from build123d import *

# Parameters (mm, degrees)
SKETCH1_W           = 65.4
SKETCH1_H           = 65.4
BOSS_EXTRUDE1_DEPTH = 1.12
FILLET1_R           = 4
BOSS_EXTRUDE2_START = 10
BOSS_EXTRUDE2_DEPTH = 10
CUT_EXTRUDE1_REACH  = 75.96
SKETCH4_W           = 19.5
SKETCH4_H           = 3.5
CUT_EXTRUDE2_DEPTH  = 2.5
FILLET3_R           = 2
SKETCH5_W           = 1.6
SKETCH5_H           = 49.8
SKETCH5_W_2         = 49.8
SKETCH5_H_2         = 1.6
BOSS_EXTRUDE3_DEPTH = 1
BOSS_EXTRUDE4_DEPTH = 3.8
SKETCH7_R           = 1.4
CUT_EXTRUDE3_DEPTH  = 11.12
SKETCH8_R           = 2.75
CUT_EXTRUDE4_DEPTH  = 4
FILLET4_R           = 1.5
FILLET5_R           = 1.5


with BuildPart() as part:
    # Sketch1 → Boss-Extrude1 (new body)
    with BuildSketch(Plane(origin=(0, 0, 0), x_dir=(1, 0, 0), z_dir=(0, 1, 0))):
        Rectangle(SKETCH1_W, SKETCH1_H)
    extrude(amount=BOSS_EXTRUDE1_DEPTH)

    # Fillet1
    fillet1_edges = [part.edges().sort_by_distance(p)[0] for p in [
        (32.7, 0.56, 32.7),
        (-32.7, 0.56, 32.7),
        (-32.7, 0.56, -32.7),
        (32.7, 0.56, -32.7),
    ]]
    fillet(fillet1_edges, radius=FILLET1_R)

    # Sketch2 → Boss-Extrude2 (add)
    with BuildSketch(Plane(origin=(0, 1.12, 0), x_dir=(1, 0, 0), z_dir=(0, 1, 0)).offset(BOSS_EXTRUDE2_START)):
        with BuildLine():
            Line((-32.7, 28.7), (-32.7, -28.7))
            ThreePointArc((-32.7, -28.7), (-31.528427125, -31.528427125), (-28.7, -32.7))
            Line((-28.7, -32.7), (28.7, -32.7))
            ThreePointArc((28.7, -32.7), (31.528427125, -31.528427125), (32.7, -28.7))
            Line((32.7, -28.7), (32.7, 28.7))
            ThreePointArc((32.7, 28.7), (31.528427125, 31.528427125), (28.7, 32.7))
            Line((28.7, 32.7), (-28.7, 32.7))
            ThreePointArc((-28.7, 32.7), (-31.528427125, 31.528427125), (-32.7, 28.7))
        make_face()
        with BuildLine():
            Line((24.9, 28.7), (-24.9, 28.7))
            ThreePointArc((-24.9, 28.7), (-26.012994231, 26.012994231), (-28.7, 24.9))
            Line((-28.7, 24.9), (-28.7, -24.9))
            ThreePointArc((-28.7, -24.9), (-26.012994231, -26.012994231), (-24.9, -28.7))
            Line((-24.9, -28.7), (24.9, -28.7))
            ThreePointArc((24.9, -28.7), (26.012994231, -26.012994231), (28.7, -24.9))
            Line((28.7, -24.9), (28.7, 24.9))
            ThreePointArc((28.7, 24.9), (26.012994231, 26.012994231), (24.9, 28.7))
        make_face(mode=Mode.SUBTRACT)
    extrude(amount=-BOSS_EXTRUDE2_DEPTH)

    # Sketch3 → Cut-Extrude1 (cut, up to next)
    with BuildSketch(Plane(origin=(0, 0, -32.7), x_dir=(-1, 0, 0), z_dir=(0, 0, -1)), mode=Mode.PRIVATE) as cut_extrude1_sk1:
        with BuildLine():
            Line((-3, 6.5), (3, 6.5))
            ThreePointArc((3, 6.5), (5, 4.5), (3, 2.5))
            Line((3, 2.5), (-3, 2.5))
            ThreePointArc((-3, 2.5), (-5, 4.5), (-3, 6.5))
        make_face()
    cut_extrude1_tool1 = extrude(cut_extrude1_sk1.sketch, amount=-CUT_EXTRUDE1_REACH, mode=Mode.PRIVATE) & part.part
    add(cut_extrude1_tool1.solids().sort_by_distance((0, 4.5, -32.7))[0], mode=Mode.SUBTRACT)

    # Sketch4 → Cut-Extrude2 (cut)
    with BuildSketch(Plane.XY.offset(-28.7)):
        with Locations((0, 2.87)):
            Rectangle(SKETCH4_W, SKETCH4_H)
    extrude(amount=-CUT_EXTRUDE2_DEPTH, mode=Mode.SUBTRACT)

    # Fillet3
    # the kernel refuses this fillet: 2 mm, written as the material it takes off along each edge
    with BuildSketch(Plane(origin=(-0.003603246, 4.62, -28.7), x_dir=(0, 1, 0), z_dir=(1, 0, 0)), Plane(origin=(-9.75, 4.62, -28.7), x_dir=(0, 1, 0), z_dir=(1, 0, 0))) as fillet3_piece_1:
        with BuildLine():
            CenterArc((FILLET3_R, -FILLET3_R), FILLET3_R, 90, 90)
            Line((0, -FILLET3_R), (0, 0))
            Line((0, 0), (FILLET3_R, 0))
        make_face()
    extrude(amount=9.753603246, mode=Mode.SUBTRACT)

    # Sketch5 → Boss-Extrude3 (add)
    with BuildSketch(Plane(origin=(0, 11.12, 0), x_dir=(1, 0, 0), z_dir=(0, 1, 0))):
        with Locations((-29.5, 0)):
            Rectangle(SKETCH5_W, SKETCH5_H)
        with Locations((0, -29.5)):
            Rectangle(SKETCH5_W_2, SKETCH5_H_2)
        with Locations((29.5, 0)):
            Rectangle(SKETCH5_W, SKETCH5_H)
        with Locations((0, 29.5)):
            Rectangle(SKETCH5_W_2, SKETCH5_H_2)
    extrude(amount=BOSS_EXTRUDE3_DEPTH)

    # Sketch6 → Boss-Extrude4 (add)
    with BuildSketch(Plane(origin=(0, 1.12, 0), x_dir=(1, 0, 0), z_dir=(0, 1, 0))):
        Polygon((-9.5, -4.3), (9.5, -4.3), (9.5, 1.7), (11.5, 1.7), (11.5, -6.3), (-11.5, -6.3), (-11.5, 1.7), (-9.5, 1.7), align=None)
    extrude(amount=BOSS_EXTRUDE4_DEPTH)

    # Sketch7 → Cut-Extrude3 (cut)
    with BuildSketch(Plane(origin=(0, 11.12, 0), x_dir=(1, 0, 0), z_dir=(0, 1, 0))):
        with Locations(Location((-28.9, 28.9, 0), (0, 0, 270))):
            Circle(SKETCH7_R)
        with Locations(Location((28.9, 28.9, 0), (0, 0, 270))):
            Circle(SKETCH7_R)
        with Locations(Location((28.9, -28.9, 0), (0, 0, 270))):
            Circle(SKETCH7_R)
        with Locations(Location((-28.9, -28.9, 0), (0, 0, 270))):
            Circle(SKETCH7_R)
    extrude(amount=-CUT_EXTRUDE3_DEPTH, mode=Mode.SUBTRACT)

    # Sketch8 → Cut-Extrude4 (cut)
    with BuildSketch(Plane.XZ):
        with Locations(Location((-28.9, 28.9, 0), (0, 0, 270))):
            Circle(SKETCH8_R)
        with Locations(Location((28.9, 28.9, 0), (0, 0, 270))):
            Circle(SKETCH8_R)
        with Locations(Location((28.9, -28.9, 0), (0, 0, 270))):
            Circle(SKETCH8_R)
        with Locations(Location((-28.9, -28.9, 0), (0, 0, 270))):
            Circle(SKETCH8_R)
    extrude(amount=-CUT_EXTRUDE4_DEPTH, mode=Mode.SUBTRACT)

    # Fillet4
    fillet4_edges = [part.edges().sort_by_distance(p)[0] for p in [
        (-11.5, 1.12, 2.3),
        (0, 1.12, 6.3),
        (11.5, 1.12, 2.3),
    ]]
    fillet(fillet4_edges, radius=FILLET4_R)

    # Fillet5
    fillet5_edges = [part.edges().sort_by_distance(p)[0] for p in [
        (-17.325, 1.12, -28.7),
        (26.012994231, 1.12, -26.012994231),
        (17.325, 1.12, -28.7),
        (-26.012994231, 1.12, -26.012994231),
        (-28.7, 1.12, 0),
        (-26.012994231, 1.12, 26.012994231),
        (0, 1.12, 28.7),
        (26.012994231, 1.12, 26.012994231),
        (28.7, 1.12, 0),
    ]]
    fillet(fillet5_edges, radius=FILLET5_R)


solid = part.part
Part model, mm, in its own coordinate system. A direction names the side the tool comes from. Coordinates: 2 decimals unless noted, no trailing zeros. Loops run counter-clockwise (first coordinate to the right, second up) from the corner with the lowest first, then second, coordinate; pieces in that order, holes last. Notation, with made-up numbers: (20.25, 81) - (61.25, 81) arc R16 ccw to (61.25, 104) - close; hole circle Ø7 at (70, -30.75). An arc over 180 degrees is marked (long way). Write each question's results on one line, items separated by ' | '. Start each with the question number.
Q1. Which spindle directions (+Z, -Z, +X, -X, +Y, -Y) get a long thin tool onto all of the face, cutting with end or side? Do faces 3 (the cylindrical face through (-4.47, 6.124, -28.763)), 4 (the flat face through (0, 2.5, -32)), 5 (the flat face through (-32.7, 6, 0)), 6 (the flat face through (0, 7, 28.7)), 7 (the cylindrical face through (29.021, 1.972, 31.647)). Say none if no direction does.
Q2. Slice it at B-B on x = 21. Give the cut face in (y, z), and give its area (3 significant figures).
Q3. Probe line 1 along X through (y, z) = (9.5, -28.9) (3 decimals); line 2 along X through (y, z) = (2.6, 28.9) (3 decimals); line 3 along X through (y, z) = (11, 16). List the from-to ranges inside material, lowest first.
Q4. Slice it at C-C on z = -17. Give the cut face in (x, y), and give its area (3 significant figures).
Q5. Slice it at D-D on x = -10.5. Give the cut face in (y, z), and give its area (3 significant figures).
Q6. Two-plate mould, pull along Z, no slides. Class faces 1 (the flat face through (0, 12.12, 29)), 2 (the flat face through (11.5, 4, 2)): +Z half, -Z half, draft (parallel to the pull), parting line (faces both ways), or undercut.
Q7. Slice it at A-A on y = 8.5. Give the cut face in (x, z), and give its area (3 significant figures).
Q8. Drop flat-ended pins along their axis: pin 1 Ø2 at (x, y) = (0.5, 4.5) entering from -Z; pin 2 Ø3 at (x, z) = (-28.9, 28.9) entering from +Y; pin 3 Ø9 at (x, z) = (-4.5, 2) entering from +Y. Give the stop position or say it passes through.
Answer:
1) face 3: none | face 4: -Z | face 5: +Z, -Z, -X, +Y, -Y | face 6: +Y | face 7: -Y
2) outline: (0, -32.7) - (11.12, -32.7) - (11.12, -30.3) - (12.12, -30.3) - (12.12, -28.7) - (2.62, -28.7) arc R1.5 cw to (1.12, -27.2) - (1.12, 27.2) arc R1.5 cw to (2.62, 28.7) - (12.12, 28.7) - (12.12, 30.3) - (11.12, 30.3) - (11.12, 32.7) - (0, 32.7) - close | area: 157 mm2
3) line 1: x = -32.695 to -30.3, -27.5 to 27.5, 30.3 to 32.695 | line 2: x = -32.695 to -31.65, -26.15 to 26.15, 31.65 to 32.695 | line 3: x = -32.7 to -28.7, 28.7 to 32.7
4) outline: (-32.7, 0) - (32.7, 0) - (32.7, 11.12) - (30.3, 11.12) - (30.3, 12.12) - (28.7, 12.12) - (28.7, 2.62) arc R1.5 cw to (27.2, 1.12) - (-27.2, 1.12) arc R1.5 cw to (-28.7, 2.62) - (-28.7, 12.12) - (-30.3, 12.12) - (-30.3, 11.12) - (-32.7, 11.12) - close | area: 157 mm2
5) outline: (0, -32.7) - (11.12, -32.7) - (11.12, -30.3) - (12.12, -30.3) - (12.12, -28.7) - (2.62, -28.7) arc R1.5 cw to (1.12, -27.2) - (1.12, -1.7) - (4.92, -1.7) - (4.92, 6.3) - (2.62, 6.3) arc R1.5 cw to (1.12, 7.8) - (1.12, 27.2) arc R1.5 cw to (2.62, 28.7) - (12.12, 28.7) - (12.12, 30.3) - (11.12, 30.3) - (11.12, 32.7) - (0, 32.7) - close | area: 188 mm2
6) face 1: draft | face 2: undercut
7) outline: (-32.7, -28.7) arc R4 ccw to (-28.7, -32.7) - (28.7, -32.7) arc R4 ccw to (32.7, -28.7) - (32.7, 28.7) arc R4 ccw to (28.7, 32.7) - (-28.7, 32.7) arc R4 ccw to (-32.7, 28.7) - close; hole circle Ø2.8 at (-28.9, -28.9); hole circle Ø2.8 at (-28.9, 28.9); hole (-28.7, -24.9) arc R3.8 cw to (-24.9, -28.7) - (24.9, -28.7) arc R3.8 cw to (28.7, -24.9) - (28.7, 24.9) arc R3.8 cw to (24.9, 28.7) - (-24.9, 28.7) arc R3.8 cw to (-28.7, 24.9) - close; hole circle Ø2.8 at (28.9, -28.9); hole circle Ø2.8 at (28.9, 28.9) | area: 989 mm2
8) pin 1: stops at z = 4.3 | pin 2: stops at y = 11.12 | pin 3: stops at y = 4.92
